```python
from build123d import *

# Parameters (mm, degrees)
SKETCH_1_R          = 4.45
EXTRUDE_1_DEPTH     = 1.9
SKETCH_2_R          = 4.45
SKETCH_2_R_2        = 3.1
CUT_EXTRUDE_2_DEPTH = 1.31
SKETCH_3_R          = 1
CUT_EXTRUDE_3_DEPTH = 3.8
CHAMFER_1_SIZE      = 0.25
CHAMFER_2_SIZE      = 2
CHAMFER_2_SIZE2     = 0.15
CHAMFER_3_SIZE      = 0.15
CHAMFER_3_SIZE2     = 2.2
SKETCH_4_R          = 1.5
CUT_EXTRUDE_1_DEPTH = 10
CHAMFER_4_SIZE      = 0.1


with BuildPart() as part:
    # 草图1 → 拉伸1 (new, symmetric)
    with BuildSketch(Plane.XY):
        with Locations(Location((0, 0, 0), (0, 0, 180))):
            Circle(SKETCH_1_R)
    extrude(amount=EXTRUDE_1_DEPTH, both=True)

    # 草图2 → 拉伸2 (cut, symmetric)
    with BuildSketch(Plane.XY):
        with Locations(Location((0, 0, 0), (0, 0, 180))):
            Circle(SKETCH_2_R)
        Circle(SKETCH_2_R_2, mode=Mode.SUBTRACT)
    extrude(amount=CUT_EXTRUDE_2_DEPTH, both=True, mode=Mode.SUBTRACT)

    # 草图3 → 拉伸3 (cut)
    with BuildSketch(Plane.XY.offset(1.9)):
        Circle(SKETCH_3_R)
    extrude(amount=-CUT_EXTRUDE_3_DEPTH, mode=Mode.SUBTRACT)

    # 倒角1
    chamfer_1_edges = [part.edges().sort_by_distance(p)[0] for p in [
        (-1, 0, 1.9),
        (-1, 0, -1.9),
    ]]
    chamfer(chamfer_1_edges, length=CHAMFER_1_SIZE)

    # 倒角2
    chamfer_2_edges = [part.edges().sort_by_distance(p)[0] for p in [
        (4.45, 0, -1.9),
    ]]
    chamfer_2_side = [part.faces().sort_by_distance(p)[0] for p in [
        (-1.375865007, 0, -1.9),
    ]]
    chamfer(chamfer_2_edges, length=CHAMFER_2_SIZE, length2=CHAMFER_2_SIZE2, reference=chamfer_2_side[0])

    # 倒角3
    chamfer_3_edges = [part.edges().sort_by_distance(p)[0] for p in [
        (4.45, 0, 1.9),
    ]]
    chamfer_3_side = [part.faces().sort_by_distance(p)[0] for p in [
        (4.45, 0, 1.605),
    ]]
    chamfer(chamfer_3_edges, length=CHAMFER_3_SIZE, length2=CHAMFER_3_SIZE2, reference=chamfer_3_side[0])

    # 草图4 → 切除-拉伸1 (cut)
    with BuildSketch(Plane(origin=(0, 0, -1.9), x_dir=(-1, 0, 0), z_dir=(0, 0, -1))):
        Circle(SKETCH_4_R)
    extrude(amount=-CUT_EXTRUDE_1_DEPTH, mode=Mode.SUBTRACT)

    # 倒角4
    chamfer_4_edges = [part.edges().sort_by_distance(p)[0] for p in [
        (1.5, 0, 1.9),
        (1.5, 0, -1.9),
    ]]
    chamfer(chamfer_4_edges, length=CHAMFER_4_SIZE)


solid = part.part
```
CAD build for the part. Positions are in the model's coordinates, mm. A direction names the side the tool comes from. Give positions to 0.01 mm unless a question says otherwise; leave off trailing zeros. Write each loop counter-clockwise with the first axis right and the second up, starting at its lowest first coordinate (ties: lowest second). Pieces come first, ordered by that corner, then holes. Notation, with made-up numbers: M 22,-34.75 L 70,-34.75 A4 cw 70,-28.75 Z; hole C 38,48 d8. An arc over 180 degrees is marked long. Return JSON: item names as keys, results as strings. Group by question number.
(1) Band-saw the part on A-A (x = 0). Give the cut face in (y, z), and give its area (3 significant figures).
(2) 3-axis set-ups, long thin cutter, end or side, ignore diameter. For faces 1 (the face through (-2, 3, -1.31)), 2 (the face through (3.28, -3.01, 1.53)): which of +Z, -Z, +X, -X, +Y, -Y reach the whole face in a straight line?
(3) Flat gauge pin, fed straight in: pin 1 Ø3 at (x, y) = (-3.5, 2.5) entering from -Z. Where does the tip first touch, or does it go through?
(4) Mould opens along X. For faces 3 (the face through (-2, 3, 1.31)), 4 (the face through (1.5, 0.07, -0.03)), 5 (the face through (1.43, -2.75, -0.02)) say: pulls with the +X half, pulls with the -X half, needs draft (parallel to the pull), parting line crosses it, or undercut.
(5) Band-saw the part on C-C (z = 1.55). Give the cut face in (x, y), and give its area (3 significant figures).
(6) Drill centre lines: L1, parallel to Y at x = 0, z = -0.05; L2, parallel to Y at x = 0, z = -1.5; L3, parallel to Z at x = -2.5, y = 2. Where is each one in solid material? Low to high. Write a range as [from, to].
Entries:
{
 "1": {"outline": "M -4.45,-1.75 L -2.45,-1.9 L -1.6,-1.9 L -1.5,-1.8 L -1.5,1.8 L -1.6,1.9 L -2.25,1.9 L -4.45,1.75 L -4.45,1.31 L -3.1,1.31 L -3.1,-1.31 L -4.45,-1.31 Z; M 1.5,-1.8 L 1.6,-1.9 L 2.45,-1.9 L 4.45,-1.75 L 4.45,-1.31 L 3.1,-1.31 L 3.1,1.31 L 4.45,1.31 L 4.45,1.75 L 2.25,1.9 L 1.6,1.9 L 1.5,1.8 Z", "area": "14.7 mm^2"},
 "2": {"face 1": "none", "face 2": "+Z, -Z"},
 "3": {"pin 1": "stops at z = -1.87"},
 "4": {"face 3": "needs draft", "face 4": "undercut", "face 5": "parting line crosses it"},
 "5": {"outline": "C 0,0 d8.9; hole C 0,0 d3", "area": "55.1 mm^2"},
 "6": {"L1": "y = [-3.1, -1.5], [1.5, 3.1]", "L2": "y = [-4.45, -1.5], [1.5, 4.45]", "L3": "z = [-1.84, -1.31], [1.31, 1.84]"}
}
